```python
from build123d import *

# Parameters (mm, degrees)
SKETCH_1_W          = 48
SKETCH_1_H          = 8
EXTRUDE_1_DEPTH     = 6
SKETCH_2_R          = 1.65
CUT_EXTRUDE_1_DEPTH = 15
FILLET_1_R          = 4


with BuildPart() as part:
    # 草图1 → 凸台-拉伸1 (new body)
    with BuildSketch(Plane(origin=(0, 0, 0), x_dir=(1, 0, 0), z_dir=(0, 1, 0))):
        Rectangle(SKETCH_1_W, SKETCH_1_H)
    extrude(amount=EXTRUDE_1_DEPTH)

    # 草图2 → 切除-拉伸1 (cut)
    with BuildSketch(Plane(origin=(0, 6, 0), x_dir=(1, 0, 0), z_dir=(0, 1, 0))):
        with Locations(Location((20, 0, 0), (0, 0, 270))):
            Circle(SKETCH_2_R)
        with Locations(Location((-20, 0, 0), (0, 0, 270))):
            Circle(SKETCH_2_R)
    extrude(amount=-CUT_EXTRUDE_1_DEPTH, mode=Mode.SUBTRACT)

    # 圆角1
    fillet_1_edges = [part.edges().sort_by_distance(p)[0] for p in [
        (-24, 3, 4),
        (-24, 3, -4),
        (24, 3, -4),
        (24, 3, 4),
    ]]
    fillet(fillet_1_edges, radius=FILLET_1_R - 0.0001)  # a hair under: the kernel refuses the full size


solid = part.part
```
Here's how the part is built. I have some questions about the finished solid (model axes, mm). Coordinates: 2 decimals unless noted, no trailing zeros. Order: outer loops, then holes, each group sorted by start corner. A loop starts at its lowest first (then second) coordinate and runs counter-clockwise, first axis right, second up. Notation, with made-up numbers: (44.5, 6.5) -> (69.5, 6.5) arc R20 cw to (69.5, 18.5) -> close; hole circle Ø6 at (46.25, -8.75). An arc over 180 degrees is marked (long way). Return JSON: item names as keys, results as strings.
1) I'm going to push a flat-ended pin straight in: P1, Ø4, axis at x = 20, z = 0, coming from the -Y side. Where does the tip first touch, or does it pass through?
Conclusion:
{"P1": "stops at y = 0"}
2) If we section it at A-A on y = 0.95: State how many separate pieces and enclosed holes the cut face has, plus the area to 3 significant figures.
Conclusion:
{"separate pieces": "1", "enclosed holes": "2", "area": "353 mm²"}
3) If we section it at C-C on z = -2.5: List the corners of the cut face in (x, y) for me, plus the area to 3 significant figures.
Conclusion:
{"outline": "(-23.12, 0) -> (23.12, 0) -> (23.12, 6) -> (-23.12, 6) -> close", "area": "277 mm²"}
4) Thinking about a two-plate mould opening in X: for faces 1 (the cylindrical face through (22.797, 3.042, 2.859)), 2 (the cylindrical face through (21.636, 3.042, -0.215)), 3 (the flat face through (0, 3, 4)), 4 (the cylindrical face through (-18.364, 3.042, -0.215)), which applies, +X half, -X half, draft (parallel to the pull), parting line (faces both ways), or undercut?
Conclusion:
{"face 1": "+X half", "face 2": "undercut", "face 3": "draft", "face 4": "undercut"}
5) If we section it at D-D on z = 2.75: List the corners of the cut face in (x, y) for me, plus the area to 3 significant figures.
Conclusion:
{"outline": "(-22.9, 0) -> (22.9, 0) -> (22.9, 6) -> (-22.9, 6) -> close", "area": "275 mm²"}
6) If I drill on probe 1 along X at (y, z) = (3.7, 0); probe 2 along X at (y, z) = (3.25, -0.75); probe 3 along Z at (x, y) = (19, 3.1), over which ranges is the centre line in solid material (lowest first)?
Conclusion:
{"probe 1": "x = -24 to -21.65, -18.35 to 18.35, 21.65 to 24", "probe 2": "x = -23.93 to -21.47, -18.53 to 18.53, 21.47 to 23.93", "probe 3": "z = -4 to -1.31, 1.31 to 4"}
7) If we section it at B-B on z = -0.75: List the corners of the cut face in (x, y) for me, plus the area to 3 significant figures.
Conclusion:
{"outline": "(-23.93, 0) -> (-21.47, 0) -> (-21.47, 6) -> (-23.93, 6) -> close; (-18.53, 0) -> (18.53, 0) -> (18.53, 6) -> (-18.53, 6) -> close; (21.47, 0) -> (23.93, 0) -> (23.93, 6) -> (21.47, 6) -> close", "area": "252 mm²"}
